Source: CAD feature listing. Evaluate the final solid. Frame: model axes, mm. Round coordinates to 2 decimals unless told otherwise and drop trailing zeros. Loops run counter-clockwise (first coordinate to the right, second up) from the corner with the lowest first, then second, coordinate; pieces in that order, holes last. Notation, with made-up numbers: M 22,13 L 54,13 A16 ccw 54,22 Z; hole C 58,43 d2. An arc over 180 degrees is marked long. One line per item, written item: value.
from build123d import *

# Parameters (mm, degrees)
F0_W             = 406.4
F0_H             = 660.4
F1_DEPTH         = 11.1125
F2_W             = 38.1
F2_H             = 88.9
F3_DEPTH         = 25.4
F3_COPIES2_COUNT = 2


# Not quite as in the source:
# - a pattern or mirror of a feature is missing from the dataset's text; its kind, count and spacing are read off the source's solid


with BuildPart() as f1:
    # F0 (on Top) → F1 (new body)
    with BuildSketch(Plane.XY):
        Rectangle(F0_W, F0_H)
    extrude(amount=F1_DEPTH)

    # F2 (on face) → F3 (cut)
    with BuildSketch(Plane.XY.offset(11.1125)):
        with Locations((-184.15, -285.75)):
            Rectangle(F2_W, F2_H)
    f3 = extrude(amount=-F3_DEPTH, mode=Mode.SUBTRACT)

    # F3_copies: F3 across plane
    add(f3.mirror(Plane(origin=(0, 0, 0), x_dir=(0, 0, 1), z_dir=(1, 0, 0))), mode=Mode.SUBTRACT)

    # F3_copies1: F3 across plane
    add(f3.mirror(Plane.ZX), mode=Mode.SUBTRACT)

    # F3_copies2: F3 ×2 about axis
    f3_copies2_axis = Axis((0, 0, 0), (0, 0, 1))
    for i in range(1, F3_COPIES2_COUNT):
        add(f3.rotate(f3_copies2_axis, i * 360 / F3_COPIES2_COUNT), mode=Mode.SUBTRACT)


solid = f1.part
1. Section query A-A (z = 5.25). Return the cut outline in (x, y), and give its area (3 significant figures).
Report:
outline: M -203.2,-241.3 L -165.1,-241.3 L -165.1,-330.2 L 165.1,-330.2 L 165.1,-241.3 L 203.2,-241.3 L 203.2,241.3 L 165.1,241.3 L 165.1,330.2 L -165.1,330.2 L -165.1,241.3 L -203.2,241.3 Z
area: 255,000 mm2
2. Ray query, line 1 (X direction, y = -272, z = 7.75). Return the intervals inside material, ascending. Write a range as [from, to].
Report:
line 1: x = [-165.1, 165.1]
3. Pin query (flat end, axial travel): pin 1 (3.5 mm diameter, centred on y = 288.5, z = 8, fed in from +X); pin 2 (5.5 mm diameter, centred on x = 180, z = 8, fed in from -Y); pin 3 (3.5 mm diameter, centred on x = 192, z = 7.5, fed in from +Y). Return the tip coordinate at first contact, or that it passes through.
Report:
pin 1: stops at x = 165.1
pin 2: stops at y = -241.3
pin 3: stops at y = 241.3
4. Section query B-B (y = 282.5). Return the cut outline in (x, z), and give its area (3 significant figures).
Report:
outline: M -165.1,0 L 165.1,0 L 165.1,11.11 L -165.1,11.11 Z
area: 3,670 mm2
